```python
from build123d import *

# Parameters (mm, degrees)
F0_R     = 7.5
F1_DEPTH = 10
F0_R_2   = 12.5
F2_DEPTH = 4.8
F3_D     = 6.2
F3_DEPTH = 10
F3_TIP   = 1.862667919
F4_D     = 10.2
F4_DEPTH = 6.5
F4_TIP   = 3.064389157


with BuildPart() as f1:
    # F0 (on Top) → F1 (new body)
    with BuildSketch(Plane.XY):
        Circle(F0_R)
    extrude(amount=F1_DEPTH)

    # F0 (on Top) → F2 (join)
    with BuildSketch(Plane.XY):
        Circle(F0_R_2)
        Circle(F0_R, mode=Mode.SUBTRACT)
    extrude(amount=F2_DEPTH)

    # F3
    with Locations(Plane(origin=(0, 0, 0), x_dir=(1, 0, 0), z_dir=(0, 0, -1))):
        with Locations((0, 0)):
            Hole(F3_D / 2, depth=F3_DEPTH)
            with Locations((0, 0, -(F3_DEPTH + F3_TIP / 2))):  # 118° drill point
                Cone(0, F3_D / 2, F3_TIP, mode=Mode.SUBTRACT)

    # F4
    with Locations(Plane(origin=(0, 0, 0), x_dir=(1, 0, 0), z_dir=(0, 0, -1))):
        with Locations((0, 0)):
            Hole(F4_D / 2, depth=F4_DEPTH)
            with Locations((0, 0, -(F4_DEPTH + F4_TIP / 2))):  # 118° drill point
                Cone(0, F4_D / 2, F4_TIP, mode=Mode.SUBTRACT)


solid = f1.part
```
The listing builds one solid part. Answer for the finished solid, in the listing's coordinates (mm). A direction names the side the tool comes from. Round coordinates to 2 decimals unless told otherwise and drop trailing zeros. Write each loop counter-clockwise with the first axis right and the second up, starting at its lowest first coordinate (ties: lowest second). Pieces come first, ordered by that corner, then holes. Notation, with made-up numbers: (87.25, 74) -> (127.25, 74) arc R32 cw to (127.25, 111) -> close; hole circle Ø4 at (-34, 0). An arc over 180 degrees is marked (long way). Answer as a JSON object with one key per item and string values. Group by question number.
Q1. Determine the mould class of faces 4 (the face through (-1.43, 2.75, 8.87)), 5 (the face through (-7.493, 0.33, 7.364)), 6 (the face through (-0.2, -5.4, 0)) for opening direction X: pulls with the +X half, pulls with the -X half, needs draft (parallel to the pull), parting line crosses it, or undercut.
Q2. Straight lines are drawn through the part: line 1 along Y through (x, z) = (0, 9.5); line 2 along Y through (x, z) = (0, 3.25); line 3 along X through (y, z) = (2.75, 5.25). For each, find the intervals that lie inside material, in ascending order.
Q3. Section D-D (y = 5.5) is taken. Write down the section's boundary in (x, z), plus the area to 3 significant figures.
Q4. Each of these flat-tipped pins is pushed along its axis until it touches: pin 1 Ø4 at (x, z) = (-5.5, 4) entering from -Y; pin 2 Ø4 at (x, z) = (7, 2) entering from -Y; pin 3 Ø1 at (y, z) = (2.5, 2) entering from -X; pin 4 Ø5 at (x, y) = (0, 0) entering from +Z. Where does it stop, or does it pass through?
Q5. Section A-A (x = 0) is taken. Write down the section's boundary in (y, z).
Q6. Which of the six approach directions +Z, -Z, +X, -X, +Y, -Y give full straight-line access (tool end or side, diameter ignored) to faces 1 (the face through (-2.4, 4.5, 3.3)), 2 (the face through (11.923, 3.755, 2.366)), 3 (the face through (0, -8, 4.8))?
Q7. Section C-C (z = 3) is taken. Write down the section's boundary in (x, y).
Check values:
{
 "1": {"face 4": "undercut", "face 5": "parting line crosses it", "face 6": "needs draft"},
 "2": {"line 1": "-7.5 to -3.1, 3.1 to 7.5", "line 2": "-12.5 to -5.1, 5.1 to 12.5", "line 3": "-6.98 to -4.3, 4.3 to 6.98"},
 "3": {"outline": "(-11.22, 0) -> (11.22, 0) -> (11.22, 4.8) -> (5.1, 4.8) -> (5.1, 10) -> (-5.1, 10) -> (-5.1, 4.8) -> (-11.22, 4.8) -> close", "area": "161 mm^2"},
 "4": {"pin 1": "y = -12", "pin 2": "y = -11.46", "pin 3": "x = -12.34", "pin 4": "through"},
 "5": {"outline": "(-12.5, 0) -> (-5.1, 0) -> (-5.1, 6.5) -> (-3.1, 7.7) -> (-3.1, 10) -> (-7.5, 10) -> (-7.5, 4.8) -> (-12.5, 4.8) -> close; (3.1, 7.7) -> (5.1, 6.5) -> (5.1, 0) -> (12.5, 0) -> (12.5, 4.8) -> (7.5, 4.8) -> (7.5, 10) -> (3.1, 10) -> close"},
 "6": {"face 1": "-Z", "face 2": "+Z, -Z", "face 3": "+Z"},
 "7": {"outline": "circle Ø25 at (0, 0); hole circle Ø10.2 at (0, 0)"}
}
